from build123d import *

# Parameters (mm, degrees)
ESBO_O6_R             = 6
CORTE_EXTRUS_O3_DEPTH = 41
ESBO_O7_R             = 1.5
CORTE_EXTRUS_O4_DEPTH = 41
CORTE_EXTRUS_O6_DEPTH = 4
ESBO_O10_W            = 50.246941072
ESBO_O10_H            = 50.246941072
CORTE_EXTRUS_O7_DEPTH = 3


with BuildPart() as part:
    # Esboço5 → Revolução1 (revolve)
    with BuildSketch(Plane.XY):
        Polygon((0, 0), (0, 40), (12, 40), (12, 20), (28, 20), (28, 40), (40, 40), (40, 0), align=None)
    revolve(axis=Axis((40, 0, 0), (-1, 0, 0)))

    # Esboço6 → Corte-extrusão3 (cut, through all)
    with BuildSketch(Plane.ZY):
        Circle(ESBO_O6_R)
        with BuildLine():
            Line((0, 7.5), (-1.5, 7.5))
            Line((-1.5, 7.5), (-1.5, 5.809475019))
            ThreePointArc((-1.5, 5.809475019), (0, 6), (1.5, 5.809475019))
            Line((1.5, 5.809475019), (1.5, 7.5))
            Line((1.5, 7.5), (0, 7.5))
        make_face()
    extrude(amount=-CORTE_EXTRUS_O3_DEPTH, mode=Mode.SUBTRACT)

    # Esboço7 → Corte-extrusão4 (cut, through all)
    with BuildSketch(Plane.ZY):
        with Locations((0, 13.001726509)):
            Circle(ESBO_O7_R)
        with Locations((13.001726509, 0)):
            Circle(ESBO_O7_R)
        with Locations((0, -13.001726509)):
            Circle(ESBO_O7_R)
        with Locations((-13.001726509, 0)):
            Circle(ESBO_O7_R)
    extrude(amount=-CORTE_EXTRUS_O4_DEPTH, mode=Mode.SUBTRACT)

    # Esboço9 → Corte-extrusão6 (cut)
    with BuildSketch(Plane.ZY):
        Polygon((0, -32.845160811), (32.845160811, 0), (0, 32.845160811), (-32.845160811, 0), align=None)
    extrude(amount=-CORTE_EXTRUS_O6_DEPTH, mode=Mode.SUBTRACT)

    # Esboço10 → Corte-extrusão7 (cut)
    with BuildSketch(Plane.ZY):
        Rectangle(ESBO_O10_W, ESBO_O10_H)
    extrude(amount=-CORTE_EXTRUS_O7_DEPTH, mode=Mode.SUBTRACT)


solid = part.part
Work out the finished part from the listing and answer in its coordinate system (mm). A direction names the side the tool comes from. Round coordinates to 2 decimals unless told otherwise and drop trailing zeros. Write each loop counter-clockwise with the first axis right and the second up, starting at its lowest first coordinate (ties: lowest second). Pieces come first, ordered by that corner, then holes. Notation, with made-up numbers: (87.5, 61.25) - (128.5, 61.25) arc R15 cw to (128.5, 73.25) - close; hole circle Ø6 at (-22.5, 11). An arc over 180 degrees is marked (long way). Answer in a Markdown table with one row per item. Add a question column.
1. A cutting plane is placed at B-B, the plane y = -5. Determine the outline of the cut face in (x, z).
2. A cutting plane is placed at C-C, the plane z = -21. Determine the outline of the cut face in (x, y).
3. The mould has two halves that part along Z. Classify faces 4 (the cylindrical face through (6.08, -8.67, 39.05)), 5 (the flat face through (3, 18, -18)), 6 (the flat face through (40, 8, -1)): +Z half, -Z half, draft (parallel to the pull), parting line (faces both ways), or undercut.
4. A cutting plane is placed at A-A, the plane x = 37. Determine the outline of the cut face in (y, z), and give its area (3 significant figures).
5. Find the intervals of material crossed by line 1 along Y through (x, z) = (20.5, 0); line 2 along X through (y, z) = (-34, -10); line 3 along X through (y, z) = (25.5, -5), in increasing order. Write a range as from..to.
6. For faces 1 (the flat face through (1, 16, 25.123)), 2 (the cylindrical face through (22, -6, 0)), 3 (the flat face through (12, -9.4, -18.3)), determine the directions among +Z, -Z, +X, -X, +Y, -Y from which every point of the face is accessible in a straight line to the end or side of a thin tool.
7. Given pin 1 (1.8 mm diameter, centred on y = 0, z = -13, fed in from +X); pin 2 (5 mm diameter, centred on x = 35.5, y = -26, fed in from +Z); pin 3 (1.5 mm diameter, centred on x = 14.5, z = 0.5, fed in from -Y); pin 4 (1.5 mm diameter, centred on x = 2, y = -14.5, fed in from +Z), each flat-ended and moving along its own axis, determine where each tip first touches the part or whether it passes through.
8. A cutting plane is placed at D-D, the plane z = -9. Determine the outline of the cut face in (x, y).
Worked out:
| question | item | result |
|---|---|---|
| 1 | outline | (0, -39.69) - (12, -39.69) - (12, -19.36) - (28, -19.36) - (28, -39.69) - (40, -39.69) - (40, -3.32) - (4, -3.32) - (4, -27.85) - (0, -27.85) - close; (0, 27.85) - (4, 27.85) - (4, 3.32) - (40, 3.32) - (40, 39.69) - (28, 39.69) - (28, 19.36) - (12, 19.36) - (12, 39.69) - (0, 39.69) - close |
| 2 | outline | (0, -34.04) - (12, -34.04) - (12, 34.04) - (0, 34.04) - (0, 25.12) - (3, 25.12) - (3, 11.85) - (4, 11.85) - (4, -11.85) - (3, -11.85) - (3, -25.12) - (0, -25.12) - close; (28, -34.04) - (40, -34.04) - (40, 34.04) - (28, 34.04) - close |
| 3 | face 4 | parting line |
| 3 | face 5 | undercut |
| 3 | face 6 | draft |
| 4 | outline | circle Ø80 at (0, 0); hole circle Ø3 at (-13, 0); hole circle Ø3 at (0, -13); hole circle Ø3 at (0, 13); hole (5.81, -1.5) - (7.5, -1.5) - (7.5, 1.5) - (5.81, 1.5) arc R6 ccw (long way) to start; hole circle Ø3 at (13, 0) |
| 4 | area | 4,880 mm^2 |
| 5 | line 1 | -20..-14.5, -11.5..-6, 7.5..11.5, 14.5..20 |
| 5 | line 2 | 0..12, 28..40 |
| 5 | line 3 | 4..12, 28..40 |
| 6 | face 1 | -X |
| 6 | face 2 | +X, -X |
| 6 | face 3 | none |
| 7 | pin 1 | through |
| 7 | pin 2 | z = 32.37 |
| 7 | pin 3 | y = -20 |
| 7 | pin 4 | z = 37.56 |
| 8 | outline | (0, -38.97) - (12, -38.97) - (12, -17.86) - (28, -17.86) - (28, -38.97) - (40, -38.97) - (40, 38.97) - (28, 38.97) - (28, 17.86) - (12, 17.86) - (12, 38.97) - (0, 38.97) - (0, 25.12) - (3, 25.12) - (3, 23.85) - (4, 23.85) - (4, -23.85) - (3, -23.85) - (3, -25.12) - (0, -25.12) - close |
